Geometry check sheet. Reference: the model listing, model coordinates, mm. A direction names the side the tool comes from. Round coordinates to 2 decimals unless told otherwise and drop trailing zeros. Write each loop counter-clockwise with the first axis right and the second up, starting at its lowest first coordinate (ties: lowest second). Pieces come first, ordered by that corner, then holes. Notation, with made-up numbers: M 28,-9.75 L 80,-9.75 A17 ccw 80,20.25 Z; hole C 56,5.5 d1. An arc over 180 degrees is marked long. Answer in a Markdown table with one row per item. Add a question column.
from build123d import *

# Parameters (mm, degrees)
F0_R     = 9.96
F1_DEPTH = 100
F2_R     = 3.25
F3_DEPTH = 25
F5_DEPTH = 6.5


with BuildPart() as f1:
    # F0 (on Top) → F1 (new body)
    with BuildSketch(Plane.XY):
        Circle(F0_R)
    extrude(amount=F1_DEPTH)

    # F2 (on face) → F3 (cut)
    with BuildSketch(Plane.XY.offset(100)):
        Circle(F2_R)
    extrude(amount=-F3_DEPTH, mode=Mode.SUBTRACT)

    # F4 (on face) → F5 (cut)
    with BuildSketch(Plane.XY.offset(100)):
        Polygon((5.10955, 2.95), (0, 5.9), (-5.10955, 2.95), (-5.10955, -2.95), (0, -5.9), (5.10955, -2.95), align=None)
    extrude(amount=-F5_DEPTH, mode=Mode.SUBTRACT)


solid = f1.part
Item 1: Section check D-D, the plane z = 69.5. Record the boundary of the cut face in (x, y), and give its area (3 significant figures).
Item 2: Section check C-C, the plane z = 80. Record the boundary of the cut face in (x, y).
Item 3: Section check B-B, the plane x = 2. Record the boundary of the cut face in (y, z), and give its area (3 significant figures).
Item 4: Gauge pin test, flat ends, axial feed: pin 1 Ø5 at (x, y) = (0.5, -1) entering from +Z; pin 2 Ø5 at (y, z) = (4.5, 39.5) entering from +X; pin 3 Ø1.8 at (y, z) = (1.5, 95) entering from -X. Record the tip position at first contact, or that the pin passes through.
Item 5: Access from +Z, -Z, +X, -X, +Y, -Y to the whole of each face (thin tool, end or side, straight path). Record for faces 1 (the flat face through (0, 0, 0)), 2 (the flat face through (-2, -3, 93.5)).
Item 6: Scan lines: probe 1 along Y at (x, z) = (0, 80); probe 2 along Z at (x, y) = (1, 1.75); probe 3 along Y at (x, z) = (-4.25, 76). Record each from-to range of solid material in increasing order. Write a range as from..to.
Item 7: Section check A-A, the plane y = 0. Record the boundary of the cut face in (x, z).
Item 8: Mould release check, pull along X, two halves, no side actions. Record for faces 3 (the flat face through (0, 0, 75)), 4 (the cylindrical face through (-7.904, -6.061, 49.3)), 5 (the flat face through (-2, 5, 100)), 6 (the flat face through (-5.11, 0, 97)): +X half, -X half, draft (parallel to the pull), parting line (faces both ways), or undercut.
Result sheet:
| question | item | result |
|---|---|---|
| 1 | outline | C 0,0 d19.92 |
| 1 | area | 312 mm^2 |
| 2 | outline | C 0,0 d19.92; hole C 0,0 d6.5 |
| 3 | outline | M -9.76,0 L 9.76,0 L 9.76,100 L 4.75,100 L 4.75,93.5 L 2.56,93.5 L 2.56,75 L -2.56,75 L -2.56,93.5 L -4.75,93.5 L -4.75,100 L -9.76,100 Z |
| 3 | area | 1,790 mm^2 |
| 4 | pin 1 | stops at z = 93.5 |
| 4 | pin 2 | stops at x = 9.76 |
| 4 | pin 3 | stops at x = -9.94 |
| 5 | face 1 | -Z, +X, -X, +Y, -Y |
| 5 | face 2 | +Z |
| 6 | probe 1 | y = -9.96..-3.25, 3.25..9.96 |
| 6 | probe 2 | z = 0..75 |
| 6 | probe 3 | y = -9.01..9.01 |
| 7 | outline | M -9.96,0 L 9.96,0 L 9.96,100 L 5.11,100 L 5.11,93.5 L 3.25,93.5 L 3.25,75 L -3.25,75 L -3.25,93.5 L -5.11,93.5 L -5.11,100 L -9.96,100 Z |
| 8 | face 3 | undercut |
| 8 | face 4 | parting line |
| 8 | face 5 | draft |
| 8 | face 6 | undercut |
